Part model, mm, in its own coordinate system. A direction names the side the tool comes from. Round coordinates to 2 decimals unless told otherwise and drop trailing zeros. Loops run counter-clockwise (first coordinate to the right, second up) from the corner with the lowest first, then second, coordinate; pieces in that order, holes last.
(1) Probe probe 1 along Z at (x, y) = (-14, 27) (3 decimals); probe 2 along Y at (x, z) = (-43.5, 192). List the from-to ranges inside material, lowest first.
(2) Mould opens along Z. For faces 1 (the face through (101.6, 9, 193)), 2 (the face through (-1, 9, 0)), 3 (the face through (64, 20.637, 27)) say: +Z half, -Z half, draft (parallel to the pull), parting line (faces both ways), or undercut.
(3) Flat gauge pins, fed straight in: pin 1 (3 mm diameter, centred on x = 7.5, z = 336.5, fed in from +Y); pin 2 (12 mm diameter, centred on x = -39, y = 30.5, fed in from +Z); pin 3 (4 mm diameter, centred on x = -61.5, z = 27.5, fed in from +Y). Where does each tip first touch, or does it go through?
(4) Tool access for faces 4 (the face through (1, 39, 190.5)), 5 (the face through (79.375, 39, 27)), 6 (the face through (-79.375, 39, 170)), 7 (the face through (-63, 20.637, 27)): list every direction of +Z, -Z, +X, -X, +Y, -Y with a clear straight run to the whole face (end or side of a thin tool).
(5) Cut at A-A on y = 53.5. Count the separate pieces of the cut face and the enclosed holes in it, then the cut area to 3 significant figures.
(6) Cut at C-C on z = 274.5. List the corners of the cut face in (x, y), then the cut area to 3 significant figures.
from build123d import *

# Parameters (mm, degrees)
SKETCH1_W           = 203.2
SKETCH1_H           = 381
BASE_EXTRUDE_DEPTH  = 19.05
SKETCH2_W           = 158.75
SKETCH2_H           = 41.275
BOSS_EXTRUDE1_DEPTH = 39.6875
SKETCH4_R           = 6.35
CUT_EXTRUDE1_DEPTH  = 38.1
LPATTERN1_COUNT     = 2
LPATTERN1_PITCH     = 142.875
SKETCH5_R           = 2.778125
CUT_EXTRUDE2_DEPTH  = 399.664839064


with BuildPart() as part:
    # Sketch1 → Base-Extrude (new body)
    with BuildSketch(Plane(origin=(0, 0, 0), x_dir=(1, 0, 0), z_dir=(0, 1, 0))):
        with Locations((0, -190.5)):
            Rectangle(SKETCH1_W, SKETCH1_H)
    extrude(amount=BASE_EXTRUDE_DEPTH)

    # Sketch2 → Boss-Extrude1 (add)
    with BuildSketch(Plane(origin=(0, 19.05, 0), x_dir=(-1, 0, 0), z_dir=(0, 1, 0))):
        with Locations((0, 26.9875)):
            Rectangle(SKETCH2_W, SKETCH2_H)
    boss_extrude1 = extrude(amount=BOSS_EXTRUDE1_DEPTH)

    # Sketch4 → Cut-Extrude1 (cut)
    with BuildSketch(Plane(origin=(0, 58.7375, 0), x_dir=(-1, 0, 0), z_dir=(0, 1, 0))):
        with Locations(Location((-63.5, 26.9875, 0), (0, 0, 90))):
            Circle(SKETCH4_R)
        with Locations(Location((63.5, 26.9875, 0), (0, 0, 90))):
            Circle(SKETCH4_R)
    cut_extrude1 = extrude(amount=-CUT_EXTRUDE1_DEPTH, mode=Mode.SUBTRACT)

    # LPattern1: Boss-Extrude1, Cut-Extrude1 ×2
    with Locations(*[(0, 0, i * LPATTERN1_PITCH) for i in range(1, LPATTERN1_COUNT)]):
        add(boss_extrude1)
        add(cut_extrude1, mode=Mode.SUBTRACT)

    # Sketch5 → Cut-Extrude2 (cut, through all)
    with BuildSketch(Plane.XZ):
        with Locations(Location((96.8375, 87.3125, 0), (0, 0, 270))):
            Circle(SKETCH5_R)
        with Locations(Location((96.8375, 131.7625, 0), (0, 0, 270))):
            Circle(SKETCH5_R)
        with Locations(Location((96.8375, 369.8875, 0), (0, 0, 270))):
            Circle(SKETCH5_R)
        with Locations(Location((96.8375, 325.4375, 0), (0, 0, 270))):
            Circle(SKETCH5_R)
        with Locations(Location((23.8125, 87.3125, 0), (0, 0, 270))):
            Circle(SKETCH5_R)
        with Locations(Location((23.8125, 131.7625, 0), (0, 0, 270))):
            Circle(SKETCH5_R)
        with Locations(Location((-96.8375, 325.4375, 0), (0, 0, 270))):
            Circle(SKETCH5_R)
        with Locations(Location((-96.8375, 369.8875, 0), (0, 0, 270))):
            Circle(SKETCH5_R)
        with Locations(Location((-23.8125, 369.8875, 0), (0, 0, 270))):
            Circle(SKETCH5_R)
        with Locations(Location((-23.8125, 325.4375, 0), (0, 0, 270))):
            Circle(SKETCH5_R)
        with Locations(Location((-96.8375, 87.3125, 0), (0, 0, 270))):
            Circle(SKETCH5_R)
        with Locations(Location((-96.8375, 131.7625, 0), (0, 0, 270))):
            Circle(SKETCH5_R)
        with Locations(Location((-23.8125, 131.7625, 0), (0, 0, 270))):
            Circle(SKETCH5_R)
        with Locations(Location((-23.8125, 87.3125, 0), (0, 0, 270))):
            Circle(SKETCH5_R)
        with Locations(Location((23.8125, 369.8875, 0), (0, 0, 270))):
            Circle(SKETCH5_R)
        with Locations(Location((23.8125, 325.4375, 0), (0, 0, 270))):
            Circle(SKETCH5_R)
    extrude(amount=-CUT_EXTRUDE2_DEPTH, mode=Mode.SUBTRACT)


solid = part.part
Final values:
1. probe 1: z = 6.35 to 47.625, 149.225 to 190.5
1. probe 2: y = 0 to 19.05
2. face 1: draft
2. face 2: -Z half
2. face 3: undercut
3. pin 1: stops at y = 19.05
3. pin 2: stops at z = 190.5
3. pin 3: stops at y = 20.64
4. face 4: +Z, +X, -X, +Y
4. face 5: +Z, -Z, +X, +Y
4. face 6: +Z, -Z, -X, +Y
4. face 7: +Y
5. separate pieces: 2
5. enclosed holes: 4
5. area: 12,600 mm2
6. outline: (-101.6, 0) - (101.6, 0) - (101.6, 19.05) - (-101.6, 19.05) - close
6. area: 3,870 mm2
